Verification items for the finished model (mm, model axes). A direction names the side the tool comes from. Round coordinates to 2 decimals unless told otherwise and drop trailing zeros. Order: outer loops, then holes, each group sorted by start corner. A loop starts at its lowest first (then second) coordinate and runs counter-clockwise, first axis right, second up. Notation, with made-up numbers: (-3, 28.25) -> (16, 28.25) arc R17 ccw to (16, 43.25) -> close; hole circle Ø11 at (12.5, 73). An arc over 180 degrees is marked (long way). Return JSON: item names as keys, results as strings. Group by question number.
1) Tool access check on faces 5 (the flat face through (-24, 5, -2.79)), 6 (the flat face through (-9, 6, -8.458)), 7 (the flat face through (-3.299, 5, 0)), 8 (the flat face through (-4.16, 6, -10)). Record the directions out of +Z, -Z, +X, -X, +Y, -Y that give a thin tool (end or side, any length) a straight path to the whole face; none if there is none.
2) Scan lines: L1, parallel to X at y = 5, z = -8.75; L2, parallel to X at y = 3.25, z = -5.75; L3, parallel to Z at x = -12, y = 3. Record each from-to range of solid material in increasing order.
3) Section check A-A on x = -6.5. Enter the section's corners in (y, z).
4) Draft check along Z on faces 1 (the cylindrical face through (-31.224, 7.362, -3.932)), 2 (the flat face through (-10, 5, 6.25)), 3 (the cylindrical face through (-1.6, 0.61, 5.99)), 4 (the flat face through (-38.62, 1, -3)). Enter one of: pulls with the +Z half, pulls with the -Z half, needs draft (parallel to the pull), parting line crosses it, or undercut.
5) Section check B-B on y = 7. Enter the section's corners in (x, z).
6) Section check C-C on z = 5.25. Enter the section's corners in (x, y).
7) Section check D-D on z = 2. Enter the section's corners in (x, y), plus the area to 3 significant figures.
8) Depth check by flat-ended pin: pin 1 (2 mm diameter, centred on x = -22, y = 4.5, fed in from -Z); pin 2 (8 mm diameter, centred on x = -11.5, y = 7, fed in from -Z); pin 3 (4 mm diameter, centred on x = -9.5, y = 7, fed in from +Z); pin 4 (2 mm diameter, centred on x = -1.22, z = 4.28, fed in from +Y). Enter the tip coordinate at first touch or a pass-through.
```python
from build123d import *

# Parameters (mm, degrees)
SKETCH1_W           = 43.7
SKETCH1_H           = 21
BOSS_EXTRUDE1_DEPTH = 1.2
SKETCH2_R           = 3.443854009
SKETCH2_R_2         = 3.137647978
BOSS_EXTRUDE2_DEPTH = 12.5
SKETCH3_W           = 13.022072972
SKETCH3_H           = 13.380807765
SKETCH3_W_2         = 9.398851567
SKETCH3_H_2         = 9.040116774
BOSS_EXTRUDE4_DEPTH = 7.5
SKETCH4_W           = 10.259815069
SKETCH4_H           = 3.946082718
BOSS_EXTRUDE5_DEPTH = 9.5
SKETCH5_R           = 1.112077857
BOSS_EXTRUDE6_DEPTH = 2
SKETCH6_R           = 1.75
CUT_EXTRUDE1_DEPTH  = 2


with BuildPart() as part:
    # Sketch1 → Boss-Extrude1 (new body)
    with BuildSketch(Plane(origin=(0, 0, 0), x_dir=(1, 0, 0), z_dir=(0, 1, 0))):
        with Locations((-16.769650206, 2.717901235)):
            Rectangle(SKETCH1_W, SKETCH1_H)
    extrude(amount=BOSS_EXTRUDE1_DEPTH)

    # Sketch2 → Boss-Extrude2 (add)
    with BuildSketch(Plane(origin=(0, 1.2, 0), x_dir=(1, 0, 0), z_dir=(0, 1, 0))):
        with Locations((-34.509085701, 2.897268631)):
            Circle(SKETCH2_R)
        with Locations((0.4316831, 2.4309134)):
            Circle(SKETCH2_R_2)
    extrude(amount=BOSS_EXTRUDE2_DEPTH)

    # Sketch3 → Boss-Extrude4 (add)
    with BuildSketch(Plane(origin=(0, 1.2, 0), x_dir=(1, 0, 0), z_dir=(0, 1, 0))):
        with Locations((-9.810195229, 0.439935301)):
            Rectangle(SKETCH3_W, SKETCH3_H)
        with Locations((-24.285144112, 7.30970658)):
            Rectangle(SKETCH3_W_2, SKETCH3_H_2)
    extrude(amount=BOSS_EXTRUDE4_DEPTH)

    # Sketch4 → Boss-Extrude5 (add)
    with BuildSketch(Plane(origin=(0, 1.2, 0), x_dir=(1, 0, 0), z_dir=(0, 1, 0))):
        with Locations((-9.290029779, 10.430699276)):
            Rectangle(SKETCH4_W, SKETCH4_H)
    extrude(amount=BOSS_EXTRUDE5_DEPTH)

    # Sketch5 → Boss-Extrude6 (add)
    with BuildSketch(Plane(origin=(0, 10.7, 0), x_dir=(1, 0, 0), z_dir=(0, 1, 0))):
        with Locations((-13.092618581, 11.040548423)):
            Circle(SKETCH5_R)
    extrude(amount=BOSS_EXTRUDE6_DEPTH)

    # Sketch6 → Cut-Extrude1 (cut)
    with BuildSketch(Plane(origin=(0, 1.2, 0), x_dir=(1, 0, 0), z_dir=(0, 1, 0))):
        with Locations((-32.119650206, 10.717901235)):
            Circle(SKETCH6_R)
        with Locations((-1.219650206, -4.282098765)):
            Circle(SKETCH6_R)
    extrude(amount=-CUT_EXTRUDE1_DEPTH, mode=Mode.SUBTRACT)


solid = part.part
```
Check result:
{
 "1": {"face 5": "+Z, +Y", "face 6": "+X, +Y", "face 7": "+Z, -Z, +Y", "face 8": "-Z, +X, +Y"},
 "2": {"L1": "-28.98 to -19.59, -14.42 to -4.16", "L2": "-36.44 to -32.58, -28.98 to -19.59, -16.32 to -3.3", "L3": "-12.4 to -8.46, -7.13 to 6.25"},
 "3": {"outline": "(0, -13.22) -> (1.2, -13.22) -> (1.2, -12.4) -> (10.7, -12.4) -> (10.7, -8.46) -> (1.2, -8.46) -> (1.2, -7.13) -> (8.7, -7.13) -> (8.7, 6.25) -> (1.2, 6.25) -> (1.2, 7.78) -> (0, 7.78) -> close"},
 "4": {"face 1": "parting line crosses it", "face 2": "pulls with the +Z half", "face 3": "undercut", "face 4": "needs draft"},
 "5": {"outline": "circle Ø6.89 at (-34.51, -2.9); (-28.98, -11.83) -> (-19.59, -11.83) -> (-19.59, -2.79) -> (-28.98, -2.79) -> close; (-16.32, -7.13) -> (-3.3, -7.13) -> (-3.3, 6.25) -> (-16.32, 6.25) -> close; (-14.42, -12.4) -> (-4.16, -12.4) -> (-4.16, -8.46) -> (-14.42, -8.46) -> close; circle Ø6.28 at (0.43, -2.43)"},
 "6": {"outline": "(-38.62, 0) -> (-2.68, 0) -> (-2.68, 1.2) -> (-3.3, 1.2) -> (-3.3, 8.7) -> (-16.32, 8.7) -> (-16.32, 1.2) -> (-38.62, 1.2) -> close; (0.24, 0) -> (5.08, 0) -> (5.08, 1.2) -> (0.24, 1.2) -> close"},
 "7": {"outline": "(-38.62, 0) -> (5.08, 0) -> (5.08, 1.2) -> (-3.3, 1.2) -> (-3.3, 8.7) -> (-16.32, 8.7) -> (-16.32, 1.2) -> (-38.62, 1.2) -> close", "area": "150 mm^2"},
 "8": {"pin 1": "z = -11.83", "pin 2": "z = -12.4", "pin 3": "z = 6.25", "pin 4": "through"}
}
